from build123d import *

# Parameters (mm, degrees)
IZIM2_R                     = 6
Y_KSEKLIK_EKSTR_ZYON1_DEPTH = 39
IZIM3_R                     = 2.5
KES_EKSTR_ZYON1_DEPTH       = 39
PAH2_SIZE                   = 1.5
FILLET2_R                   = 0.5


with BuildPart() as part:
    # Çizim2 → Yükseklik-Ekstrüzyon1 (new body)
    with BuildSketch(Plane.XY):
        Polygon((22, 15), (-22, 15), (-22, 7), (-20.5, 5.5), (-20.5, -9.5), (-11, -9.5), (-5.5, -15), (5.5, -15), (11, -9.5), (20.5, -9.5), (20.5, 5.5), (22, 7), align=None)
        Circle(IZIM2_R, mode=Mode.SUBTRACT)
    extrude(amount=Y_KSEKLIK_EKSTR_ZYON1_DEPTH)

    # Çizim3 → Kes-Ekstrüzyon1 (cut)
    with BuildSketch(Plane.XZ.offset(9.5)):
        with Locations((16.5, 32.5)):
            Circle(IZIM3_R)
        with Locations((-16.5, 32.5)):
            Circle(IZIM3_R)
        with Locations((-16.5, 6.5)):
            Circle(IZIM3_R)
        with Locations((16.5, 6.5)):
            Circle(IZIM3_R)
    extrude(amount=-KES_EKSTR_ZYON1_DEPTH, mode=Mode.SUBTRACT)

    # Pah2
    pah2_edges = [part.edges().sort_by_distance(p)[0] for p in [
        (-6, 0, 0),
    ]]
    chamfer(pah2_edges, length=PAH2_SIZE)

    # Fillet2
    fillet2_edges = [part.edges().sort_by_distance(p)[0] for p in [
        (14, 15, 32.5),
        (14, 15, 6.5),
        (-19, 15, 6.5),
        (-19, 15, 32.5),
    ]]
    fillet(fillet2_edges, radius=FILLET2_R)


solid = part.part
Design review of the part built by this model. Coordinates are the model's own, in mm. A direction names the side the tool comes from. Give positions to 0.01 mm unless a question says otherwise; leave off trailing zeros. Loops run counter-clockwise (first coordinate to the right, second up) from the corner with the lowest first, then second, coordinate; pieces in that order, holes last. Notation, with made-up numbers: M 30,-31 L 49,-31 A20 ccw 49,0 Z; hole C -4.75,5.25 d6. An arc over 180 degrees is marked long. Answer as a JSON object with one key per item and string values.
Item 1: We need section D-D (x = 0). State the section outline as (y, z) points, and give its area (3 significant figures).
Output values:
{"outline": "M -15,0 L -7.5,0 L -6,1.5 L -6,39 L -15,39 Z; M 6,1.5 L 7.5,0 L 15,0 L 15,39 L 6,39 Z", "area": "700 mm2"}
Item 2: Machinability: for faces 4 (the face through (-18.34, 2.33, 34.19)), 5 (the face through (20.5, -2, 19)), 6 (the face through (-16, -9.5, 19)), which of the approach directions +Z, -Z, +X, -X, +Y, -Y give a long, thin tool a straight path to every point of the face, cutting with its end or side? Answer none if there is none.
Output values:
{"face 4": "+Y, -Y", "face 5": "+Z, -Z, +X, -Y", "face 6": "+Z, -Z, -X, -Y"}
Item 3: We need section C-C (x = -16.5). State the section outline as (y, z) points.
Output values:
{"outline": "M -9.5,0 L 15,0 L 15,3.5 A0.5 ccw 14.5,4 L -9.5,4 Z; M -9.5,9 L 14.5,9 A0.5 ccw 15,9.5 L 15,29.5 A0.5 ccw 14.5,30 L -9.5,30 Z; M -9.5,35 L 14.5,35 A0.5 ccw 15,35.5 L 15,39 L -9.5,39 Z"}
Item 4: Mouldability with a two-part tool opening along Z and no side actions: class faces 1 (the face through (14, 2.3, 6.6)), 2 (the face through (0, 7, 39)), 3 (the face through (-21, 6, 19)) as pulls with the +Z half, pulls with the -Z half, needs draft (parallel to the pull), parting line crosses it, or undercut.
Output values:
{"face 1": "undercut", "face 2": "pulls with the +Z half", "face 3": "needs draft"}
Item 5: Wall thickness on line 1 along Z through (x, y) = (-16.5, 9.5); line 2 along Z through (x, y) = (16, -4.5); line 3 along Y through (x, z) = (7, 10): over which ranges is each line inside the solid? List them lowest first.
Output values:
{"line 1": "z = 0 to 4, 9 to 30, 35 to 39", "line 2": "z = 0 to 4.05, 8.95 to 30.05, 34.95 to 39", "line 3": "y = -13.5 to 15"}
Item 6: We need section A-A (y = 0). State the section outline as (x, z) points, and give its area (3 significant figures).
Output values:
{"outline": "M -20.5,0 L -7.5,0 L -6,1.5 L -6,39 L -20.5,39 Z; M 6,1.5 L 7.5,0 L 20.5,0 L 20.5,39 L 6,39 Z; hole C -16.5,6.5 d5; hole C -16.5,32.5 d5; hole C 16.5,6.5 d5; hole C 16.5,32.5 d5", "area": "1,050 mm2"}
Item 7: We need section B-B (z = 32.5). State the section outline as (x, y) points.
Output values:
{"outline": "M -22,7 L -20.5,5.5 L -20.5,-9.5 L -19,-9.5 L -19,14.5 A0.5 ccw -19.5,15 L -22,15 Z; M -14,-9.5 L -11,-9.5 L -5.5,-15 L 5.5,-15 L 11,-9.5 L 14,-9.5 L 14,14.5 A0.5 ccw 13.5,15 L -13.5,15 A0.5 ccw -14,14.5 Z; M 19,-9.5 L 20.5,-9.5 L 20.5,5.5 L 22,7 L 22,15 L 19.5,15 A0.5 ccw 19,14.5 Z; hole C 0,0 d12"}
Item 8: For P1, Ø3, axis at y = -2, z = 8.5, coming from the +X side; P2, Ø1.5, axis at y = -2, z = 29, coming from the -X side; P3, Ø5, axis at y = 5.5, z = 26, coming from the -X side; P4, Ø4, axis at x = 16.5, z = 6.5, coming from the +Y side, all flat-tipped, find the tip position at first contact; note any pin that passes through.
Output values:
{"P1": "stops at x = 20.5", "P2": "stops at x = -20.5", "P3": "stops at x = -22", "P4": "passes through"}
